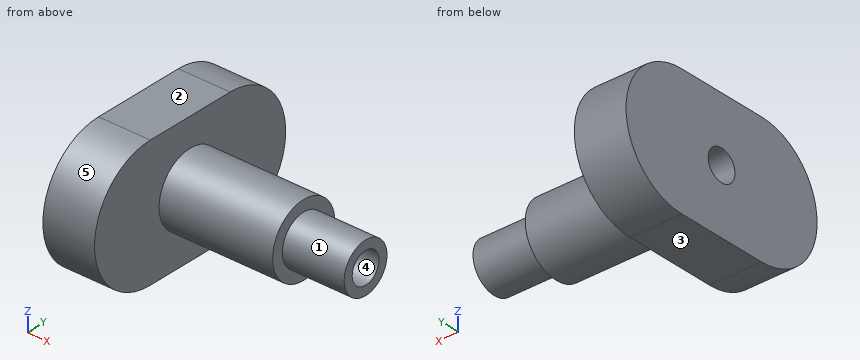
from build123d import *

# Parameters (mm, degrees)
BOSS_EXTRUDE1_DEPTH = 8.36
SKETCH2_R           = 5.8
BOSS_EXTRUDE2_DEPTH = 18.35
SKETCH3_R           = 4
BOSS_EXTRUDE3_DEPTH = 10
SKETCH4_R           = 2.5
CUT_EXTRUDE1_DEPTH  = 43.117001318


with BuildPart() as part:
    # Sketch1 → Boss-Extrude1 (new body)
    with BuildSketch(Plane.YZ):
        with BuildLine():
            Line((-7.45, 10.39), (7.45, 10.39))
            ThreePointArc((7.45, 10.39), (17.84, 0), (7.45, -10.39))
            Line((7.45, -10.39), (-7.45, -10.39))
            ThreePointArc((-7.45, -10.39), (-17.84, 0), (-7.45, 10.39))
        make_face()
    extrude(amount=BOSS_EXTRUDE1_DEPTH)

    # Sketch2 → Boss-Extrude2 (add)
    with BuildSketch(Plane.YZ.offset(8.36)):
        with Locations(Location((0, 0, 0), (0, 0, 270))):
            Circle(SKETCH2_R)
    extrude(amount=BOSS_EXTRUDE2_DEPTH)

    # Sketch3 → Boss-Extrude3 (add)
    with BuildSketch(Plane.YZ.offset(26.71)):
        with Locations(Location((0, 0, 0), (0, 0, 270))):
            Circle(SKETCH3_R)
    extrude(amount=BOSS_EXTRUDE3_DEPTH)

    # Sketch4 → Cut-Extrude1 (cut, through all)
    with BuildSketch(Plane.YZ.offset(36.71)):
        with Locations(Location((0, 0, 0), (0, 0, 270))):
            Circle(SKETCH4_R)
    extrude(amount=-CUT_EXTRUDE1_DEPTH, mode=Mode.SUBTRACT)


solid = part.part
Verification items for the finished model (mm, model axes). Face numbers are marked on the shaded views. A direction names the side the tool comes from. Give positions to 0.01 mm unless a question says otherwise; leave off trailing zeros. Order: outer loops, then holes, each group sorted by start corner. A loop starts at its lowest first (then second) coordinate and runs counter-clockwise, first axis right, second up. Notation, with made-up numbers: M 38,-24 L 90,-24 A28 ccw 90,9 Z; hole C 72.5,-21.75 d11. An arc over 180 degrees is marked long. Use one line per item in the form item = value. Start each with the question number.
Q1. Section check D-D (z = 5). Enter the section's corners in (x, y), then the cut area to 3 significant figures.
Q2. Section check A-A (y = 0). Enter the section's corners in (x, z).
Q3. Access from +Z, -Z, +X, -X, +Y, -Y to the whole of each face (thin tool, end or side, straight path). Record for the marked faces 1 and 2.
Q4. Section check B-B (z = 0). Enter the section's corners in (x, y).
Q5. Mould release check, pull along Y, two halves, no side actions. Record for the marked faces 3, 4 and 5: +Y half, -Y half, draft (parallel to the pull), parting line (faces both ways), or undercut.
Q6. Section check C-C (x = 5). Enter the section's corners in (y, z), then the cut area to 3 significant figures.
Q7. Scan lines: line 1 along Y through (x, z) = (10, 0); line 2 along X through (y, z) = (-11, -4.25); line 3 along Y through (x, z) = (12, 1.5). Record each from-to range of solid material in increasing order. Write a range as [from, to].
Q8. Go/stop test with flat-tipped pins: pin 1 Ø12 at (x, z) = (21.5, -7.5) entering from -Y; pin 2 Ø4 at (y, z) = (8.5, 5) entering from -X; pin 3 Ø4 at (y, z) = (0, 0) entering from +X; pin 4 Ø4 at (y, z) = (8, 7.5) entering from +X. Record where each tip stops, or that it passes through.
Evaluation:
q1.outline = M 0,-16.56 L 8.36,-16.56 L 8.36,-2.94 L 26.71,-2.94 L 26.71,2.94 L 8.36,2.94 L 8.36,16.56 L 0,16.56 Z
q1.area = 385 mm2
q2.outline = M 0,-10.39 L 8.36,-10.39 L 8.36,-5.8 L 26.71,-5.8 L 26.71,-4 L 36.71,-4 L 36.71,-2.5 L 0,-2.5 Z; M 0,2.5 L 36.71,2.5 L 36.71,4 L 26.71,4 L 26.71,5.8 L 8.36,5.8 L 8.36,10.39 L 0,10.39 Z
q3.face_1 = +X
q3.face_2 = +Z, +X, -X, +Y, -Y
q4.outline = M 0,-17.84 L 8.36,-17.84 L 8.36,-5.8 L 26.71,-5.8 L 26.71,-4 L 36.71,-4 L 36.71,-2.5 L 0,-2.5 Z; M 0,2.5 L 36.71,2.5 L 36.71,4 L 26.71,4 L 26.71,5.8 L 8.36,5.8 L 8.36,17.84 L 0,17.84 Z
q5.face_3 = draft
q5.face_4 = undercut
q5.face_5 = -Y half
q6.outline = M -7.45,-10.39 L 7.45,-10.39 A10.39 ccw 7.45,10.39 L -7.45,10.39 A10.39 ccw Z; hole C 0,0 d5
q6.area = 629 mm2
q7.line_1 = [-5.8, -2.5], [2.5, 5.8]
q7.line_2 = [0, 8.36]
q7.line_3 = [-5.6, -2], [2, 5.6]
q8.pin_1 = -5.6
q8.pin_2 = 0
q8.pin_3 = through
q8.pin_4 = 8.36
